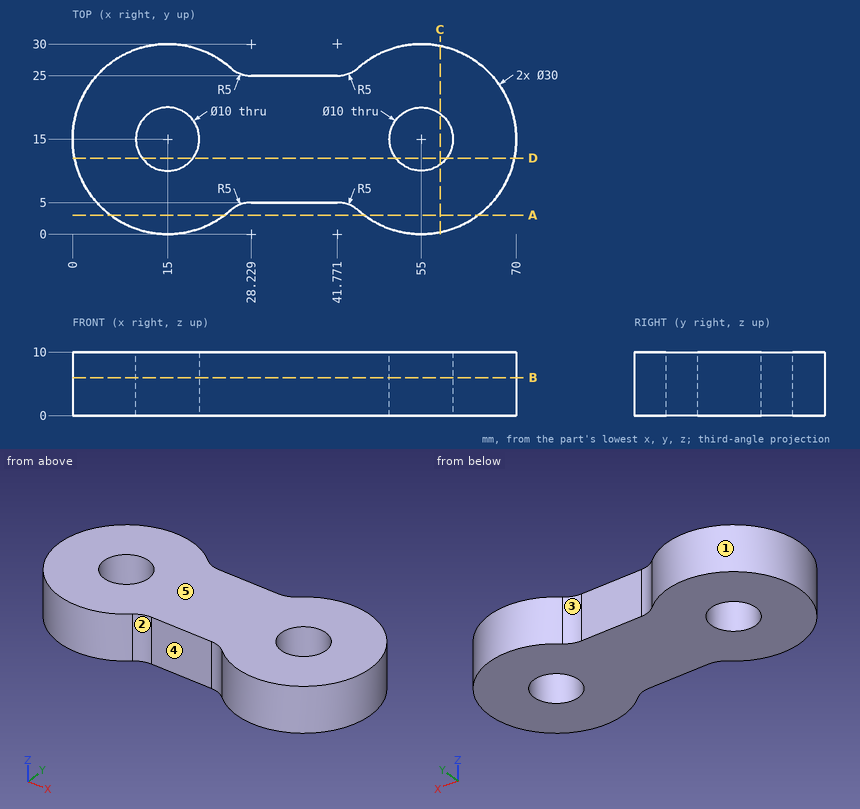
Could you check a few things on this drawing? It's one solid part, dimensions in mm from its lowest x, y, z. A direction names the side the tool comes from. Coordinates: 2 decimals unless noted, no trailing zeros. Write each loop counter-clockwise with the first axis right and the second up, starting at its lowest first coordinate (ties: lowest second). Pieces come first, ordered by that corner, then holes.
1) I'm going to push flat-ended pins straight in: pin 1 (3 mm diameter, centred on y = 21.5, z = 5.5, fed in from -X); pin 2 (3 mm diameter, centred on x = 9, z = 7.5, fed in from +Y); pin 3 (5 mm diameter, centred on x = 9, z = 6, fed in from +Y). Where does each tip first touch, or does it pass through?
Filled in:
pin 1: stops at x = 0.86
pin 2: stops at y = 29.31
pin 3: stops at y = 29.59
2) If we section it at A-A (y = 3): List the corners of the cut face in (x, z) for me.
Filled in:
outline: (6, 0) - (24, 0) - (24, 10) - (6, 10) - close; (46, 0) - (64, 0) - (64, 10) - (46, 10) - close
3) If we section it at C-C (x = 58): List the corners of the cut face in (y, z) for me, plus the area to 3 significant figures.
Filled in:
outline: (0.3, 0) - (11, 0) - (11, 10) - (0.3, 10) - close; (19, 0) - (29.7, 0) - (29.7, 10) - (19, 10) - close
area: 214 mm2
4) If we section it at D-D (y = 12): List the corners of the cut face in (x, z) for me.
Filled in:
outline: (0.3, 0) - (11, 0) - (11, 10) - (0.3, 10) - close; (19, 0) - (51, 0) - (51, 10) - (19, 10) - close; (59, 0) - (69.7, 0) - (69.7, 10) - (59, 10) - close
5) Thinking about a two-plate mould opening in X: for the marked faces 4 and 5, which applies, +X half, -X half, draft (parallel to the pull), parting line (faces both ways), or undercut?
Filled in:
face 4: undercut
face 5: draft
6) Which directions (+Z, -Z, +X, -X, +Y, -Y) give clear straight access to the entire face, cutting with the end or side of a thin tool? Please do the marked faces 1, 2 and 3.
Filled in:
face 1: +Z, -Z
face 2: +Z, -Z, -Y
face 3: +Z, -Z, +Y
7) If we section it at B-B (z = 6): List the corners of the cut face in (x, y) for me, plus the area to 3 significant figures.
Filled in:
outline: (24.92, 3.75) arc R5 cw to (28.23, 5) - (41.77, 5) arc R5 cw to (45.08, 3.75) arc R15 ccw (long way) to (45.08, 26.25) arc R5 cw to (41.77, 25) - (28.23, 25) arc R5 cw to (24.92, 26.25) arc R15 ccw (long way) to start; hole circle Ø10 at (15, 15); hole circle Ø10 at (55, 15)
area: 1,510 mm2
8) If I drill on line 1 (X direction, y = 15, z = 8.5); line 2 (Y direction, x = 15, z = 2.75); line 3 (X direction, y = 13, z = 3), over which ranges is the centre line in solid material (lowest first)?
Filled in:
line 1: x = 0 to 10, 20 to 50, 60 to 70
line 2: y = 0 to 10, 20 to 30
line 3: x = 0.13 to 10.42, 19.58 to 50.42, 59.58 to 69.87
